Could you check a few things on this model? Use its own coordinates, in mm. Face numbers are marked on the shaded views. Coordinates: 2 decimals unless noted, no trailing zeros. Loops run counter-clockwise (first coordinate to the right, second up) from the corner with the lowest first, then second, coordinate; pieces in that order, holes last.
1) Imagine slicing it at C-C on z = -55.35. Please give me the cut outline in (x, y), plus the area to 3 significant figures.
2) Imagine slicing it at D-D on x = -65.35. Please give me the cut outline in (y, z), plus the area to 3 significant figures.
3) Will these pins go through, and if not, where does the flat tip stop? P1, Ø4, axis at x = 19, y = 53, coming from the -Z side; P2, Ø8, axis at x = -65.35, z = -55.35, coming from the -Y side; P3, Ø3, axis at x = -25, z = 11.5, coming from the -Y side.
4) Imagine slicing it at B-B on z = 18. Please give me the cut outline in (x, y).
5) Thinking about a two-plate mould opening in Z: for the marked faces 1, 2 and 3, which applies, released by +Z, released by -Z, zero draft, split by the parting line, or undercut?
6) Imagine slicing it at A-A on x = 3. Please give me the cut outline in (y, z).
7) If I drill on line 1 along X through (y, z) = (98.3, -55.35); line 2 along Z through (x, y) = (-12, 98.9); line 3 along Y through (x, z) = (65.35, 58.1), over which ranges is the centre line in solid material (lowest first)?
```python
from build123d import *

# Parameters (mm, degrees)
SKETCH1_W                 = 140
SKETCH1_H                 = 120
BOSS_EXTRUDE1_DEPTH       = 100
SHELL1_T                  = -3
SKETCH6_R                 = 3.15
CUT_EXTRUDE4_DEPTH        = 3
SKETCH7_R                 = 3.15
CUT_EXTRUDE5_DEPTH        = 3
SKETCH8_W                 = 48
SKETCH8_H                 = 48
CUT_EXTRUDE6_DEPTH        = 3
SKETCH9_W                 = 5
SKETCH9_H                 = 48
BOSS_EXTRUDE2_DEPTH       = 15
SKETCH10_W                = 10
SKETCH10_H                = 48
BOSS_EXTRUDE3_DEPTH       = 3
F_3_0MM_DOWEL_HOLE1_D     = 3
F_3_0MM_DOWEL_HOLE1_DEPTH = 5
F_3_0MM_DOWEL_HOLE1_TIP   = 0.901290929


with BuildPart() as part:
    # Sketch1 → Boss-Extrude1 (new body)
    with BuildSketch(Plane(origin=(0, 0, 0), x_dir=(1, 0, 0), z_dir=(0, 1, 0))):
        Rectangle(SKETCH1_W, SKETCH1_H)
    extrude(amount=BOSS_EXTRUDE1_DEPTH)

    # Shell1
    shell1_openings = [part.faces().sort_by_distance(p)[0] for p in [
        (0, 0, 0),
        (-70, 50, 0),
        (0, 50, -60),
        (70, 50, 0),
    ]]
    offset(amount=SHELL1_T, openings=shell1_openings, kind=Kind.INTERSECTION)

    # Sketch6 → Cut-Extrude4 (cut)
    with BuildSketch(Plane.XY.offset(60)):
        with Locations((-65.35, 4.65)):
            Circle(SKETCH6_R)
        with Locations((65.35, 4.65)):
            Circle(SKETCH6_R)
    extrude(amount=-CUT_EXTRUDE4_DEPTH, mode=Mode.SUBTRACT)

    # Sketch7 → Cut-Extrude5 (cut)
    with BuildSketch(Plane(origin=(0, 100, 0), x_dir=(1, 0, 0), z_dir=(0, 1, 0))):
        with Locations(Location((-65.35, 55.35, 0), (0, 0, 270))):
            Circle(SKETCH7_R)
        with Locations(Location((65.35, 55.35, 0), (0, 0, 270))):
            Circle(SKETCH7_R)
    extrude(amount=-CUT_EXTRUDE5_DEPTH, mode=Mode.SUBTRACT)

    # Sketch8 → Cut-Extrude6 (cut)
    with BuildSketch(Plane.XZ.offset(-97)):
        Rectangle(SKETCH8_W, SKETCH8_H)
    extrude(amount=-CUT_EXTRUDE6_DEPTH, mode=Mode.SUBTRACT)

    # Sketch9 → Boss-Extrude2 (add)
    with BuildSketch(Plane.XZ.offset(-97)):
        with Locations((26.5, 0)):
            Rectangle(SKETCH9_W, SKETCH9_H)
        with Locations((-26.5, 0)):
            Rectangle(SKETCH9_W, SKETCH9_H)
    extrude(amount=BOSS_EXTRUDE2_DEPTH)

    # Sketch10 → Boss-Extrude3 (add)
    with BuildSketch(Plane.XZ.offset(-82)):
        with Locations((24, 0)):
            Rectangle(SKETCH10_W, SKETCH10_H)
        with Locations((-24, 0)):
            Rectangle(SKETCH10_W, SKETCH10_H)
    extrude(amount=BOSS_EXTRUDE3_DEPTH)

    # Ø3.0mm Dowel Hole1
    with Locations(Plane(origin=(0, 97, 0), x_dir=(-1, 0, 0), z_dir=(0, -1, 0))):
        with Locations((12, 30), (-12, 30)):
            Hole(F_3_0MM_DOWEL_HOLE1_D / 2, depth=F_3_0MM_DOWEL_HOLE1_DEPTH)
            with Locations((0, 0, -(F_3_0MM_DOWEL_HOLE1_DEPTH + F_3_0MM_DOWEL_HOLE1_TIP / 2))):  # 118° drill point
                Cone(0, F_3_0MM_DOWEL_HOLE1_D / 2, F_3_0MM_DOWEL_HOLE1_TIP, mode=Mode.SUBTRACT)


solid = part.part
```
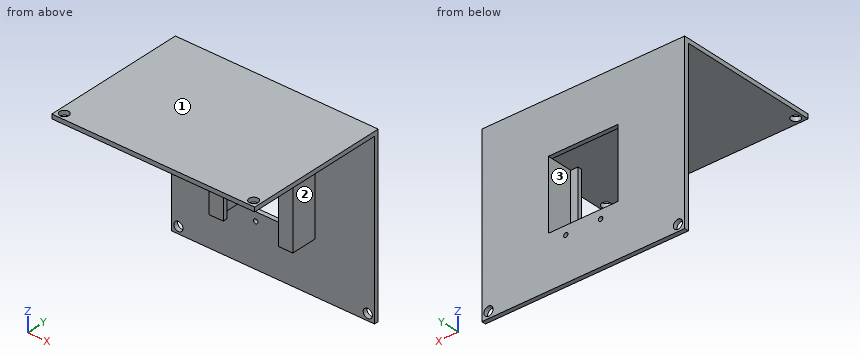
Filled in:
1. outline: (-70, 97) - (-68.5, 97) - (-68.5, 100) - (-70, 100) - close; (-62.2, 97) - (62.2, 97) - (62.2, 100) - (-62.2, 100) - close; (68.5, 97) - (70, 97) - (70, 100) - (68.5, 100) - close
1. area: 382 mm2
2. outline: (0, 57) - (1.5, 57) - (1.5, 60) - (0, 60) - close; (7.8, 57) - (97, 57) - (97, -52.2) - (100, -52.2) - (100, 60) - (7.8, 60) - close; (97, -60) - (100, -60) - (100, -58.5) - (97, -58.5) - close
2. area: 613 mm2
3. P1: stops at z = 57
3. P2: stops at y = 97
3. P3: stops at y = 79
4. outline: (-70, 97) - (-29, 97) - (-29, 79) - (-19, 79) - (-19, 82) - (-24, 82) - (-24, 100) - (-70, 100) - close; (19, 79) - (29, 79) - (29, 97) - (70, 97) - (70, 100) - (24, 100) - (24, 82) - (19, 82) - close
5. face 1: released by +Z
5. face 2: zero draft
5. face 3: undercut
6. outline: (0, 57) - (97, 57) - (97, 24) - (100, 24) - (100, 60) - (0, 60) - close; (97, -60) - (100, -60) - (100, -24) - (97, -24) - close
7. line 1: x = -70 to -68.5, -62.2 to 62.2, 68.5 to 70
7. line 2: z = -60 to -31.5, -28.5 to -24, 24 to 60
7. line 3: y = 0 to 1.5, 7.8 to 100
